from build123d import *

# Parameters (mm, degrees)
F0_R     = 10.9982
F1_DEPTH = 8.89


with BuildPart() as f1:
    # F0 (on Top) → F1 (new body)
    with BuildSketch(Plane.XY):
        with BuildLine():
            ThreePointArc((38.8529947684, 0), (28.4453239469, 28.4684513244), (0, 38.9391665957))
            ThreePointArc((0, 38.9391665957), (-27.8957339054, 28.0256688183), (-38.4710963646, 0))
            ThreePointArc((-38.4710963646, 0), (-27.9199689316, -27.9141662733), (0.0231951649, -38.3882556901))
            ThreePointArc((0.0231951649, -38.3882556901), (-9.5721699853, -15.3070070583), (13.5255, -24.8627755791))
            ThreePointArc((13.5255, -24.8627755791), (10.5110469105, -33.3749458719), (2.8113610633, -38.0928700316))
            ThreePointArc((2.8113610633, -38.0928700316), (29.4450372623, -27.1955065208), (38.8529947684, 0))
        make_face()
        with BuildLine():
            ThreePointArc((-11.4212829144, -0.1791534288), (-25.0363615935, -13.7043567881), (-38.4710963646, 0))
            ThreePointArc((-38.4710963646, 0), (-24.8572042354, 13.3460499305), (-11.4212829144, -0.1791534288))
        make_face(mode=Mode.SUBTRACT)
        Circle(F0_R, mode=Mode.SUBTRACT)
        with BuildLine():
            ThreePointArc((38.8531280306, 0.0600404714), (38.853094715, 0.0300201617), (38.8529947684, 0))
            ThreePointArc((38.8529947684, 0), (11.8021613462, 0.090060781), (38.8531280306, 0.0600404714))
        make_face(mode=Mode.SUBTRACT)
        with BuildLine():
            ThreePointArc((0, 38.9391665957), (9.8292581555, 34.8677545596), (13.9006701916, 25.0384964041))
            ThreePointArc((13.9006701916, 25.0384964041), (-9.8292581555, 15.2092382486), (0, 38.9391665957))
        make_face(mode=Mode.SUBTRACT)
        with BuildLine():
            ThreePointArc((0, 38.9391665957), (-9.8292581555, 15.2092382486), (13.9006701916, 25.0384964041))
            ThreePointArc((13.9006701916, 25.0384964041), (9.8292581555, 34.8677545596), (0, 38.9391665957))
        make_face()
        with Locations((0, 25.0384964041)):
            Circle(F0_R, mode=Mode.SUBTRACT)
        with BuildLine():
            ThreePointArc((-11.4212829144, -0.1791534288), (-24.8572042354, 13.3460499305), (-38.4710963646, 0))
            ThreePointArc((-38.4710963646, 0), (-25.0363615935, -13.7043567881), (-11.4212829144, -0.1791534288))
        make_face()
        with Locations((-24.9467829144, -0.1791534288)):
            Circle(F0_R, mode=Mode.SUBTRACT)
        with BuildLine():
            ThreePointArc((38.8531280306, 0.0600404714), (11.8021613462, 0.090060781), (38.8529947684, 0))
            ThreePointArc((38.8529947684, 0), (38.853094715, 0.0300201617), (38.8531280306, 0.0600404714))
        make_face()
        with Locations((25.3276280306, 0.0600404714)):
            Circle(F0_R, mode=Mode.SUBTRACT)
        with BuildLine():
            ThreePointArc((0.0231951649, -38.3882556901), (1.4201424448, -38.2675994791), (2.8113610633, -38.0928700316))
            ThreePointArc((2.8113610633, -38.0928700316), (10.5110469105, -33.3749458719), (13.5255, -24.8627755791))
            ThreePointArc((13.5255, -24.8627755791), (-9.5721699853, -15.3070070583), (0.0231951649, -38.3882556901))
        make_face()
        with Locations((0, -24.8627755791)):
            Circle(F0_R, mode=Mode.SUBTRACT)
        with BuildLine():
            ThreePointArc((0.0231951649, -38.3882556901), (1.4249527798, -38.3130045669), (2.8113610633, -38.0928700316))
            ThreePointArc((2.8113610633, -38.0928700316), (1.4201424448, -38.2675994791), (0.0231951649, -38.3882556901))
        make_face()
    extrude(amount=F1_DEPTH)


solid = f1.part
Can you work these out from the model? Positions are in its coordinate system, mm. Round coordinates to 2 decimals unless told otherwise and drop trailing zeros. Order: outer loops, then holes, each group sorted by start corner. A loop starts at its lowest first (then second) coordinate and runs counter-clockwise, first axis right, second up. Notation, with made-up numbers: M 36,17.5 L 93,17.5 A19 ccw 93,38.5 Z; hole C 29,63.5 d3. An arc over 180 degrees is marked long. Use a Markdown table: item, result.
1) If we mould it in two halves opening along X, with no side actions, what happens to faces 1 (the face through (5.075, -34.62, 4.383)), 2 (the face through (1.405, -38.315, 4.383)), 3 (the face through (8, -8, 0)), 4 (the face through (-14.787, -4.392, 4.383))? For each: +X half, -X half, draft (parallel to the pull), parting line (faces both ways), or undercut.
Geometry says:
| item | result |
|---|---|
| face 1 | undercut |
| face 2 | +X half |
| face 3 | draft |
| face 4 | undercut |
2) I'm going to push flat-ended pins straight in: P1, Ø1, axis at x = 25, z = 5.5, coming from the +Y side; P2, Ø1.5, axis at x = 26.5, z = 3.5, coming from the +Y side; P3, Ø5, axis at y = -24.5, z = 4, coming from the +X side. Where does each tip first touch, or does it pass through?
Geometry says:
| item | result |
|---|---|
| P1 | stops at y = 31.89 |
| P2 | stops at y = 30.91 |
| P3 | stops at x = 33.5 |
3) If I drill on line 1 along X through (y, z) = (-2, 5); line 2 along Y through (x, z) = (-5.5, 4); line 3 along X through (y, z) = (5, 0.5), over which ranges is the centre line in solid material (lowest first)?
Geometry says:
| item | result |
|---|---|
| line 1 | x = -38.54 to -35.79, -14.1 to -10.81, 10.81 to 14.52, 36.13 to 38.98 |
| line 2 | y = -38.33 to -34.39, -15.34 to -9.52, 9.52 to 15.51, 34.56 to 38.78 |
| line 3 | x = -38.42 to -34.65, -15.24 to -9.8, 9.8 to 15.5, 35.15 to 38.92 |
4) Imagine slicing it at A-A (x = 29). List the corners of the cut face in (y, z) for me.
Geometry says:
| item | result |
|---|---|
| outline | M -27.66,0 L -10.31,0 L -10.31,8.89 L -27.66,8.89 Z; M 10.43,0 L 27.9,0 L 27.9,8.89 L 10.43,8.89 Z |
5) Imagine slicing it at C-C (z = 3.25). List the corners of the cut face in (x, y) for me.
Geometry says:
| item | result |
|---|---|
| outline | M -38.47,0 A36.16 ccw 0.02,-38.39 A13.53 ccw 2.81,-38.09 A34.92 ccw 38.85,0 A36.06 ccw 0,38.94 A36.85 ccw Z; hole C -24.95,-0.18 d22; hole C 0,-24.86 d22; hole C 0,0 d22; hole C 0,25.04 d22; hole C 25.33,0.06 d22 |
6) Imagine slicing it at B-B (y = 2.5). List the corners of the cut face in (x, z) for me.
Geometry says:
| item | result |
|---|---|
| outline | M -38.53,0 L -35.61,0 L -35.61,8.89 L -38.53,8.89 Z; M -14.28,0 L -10.71,0 L -10.71,8.89 L -14.28,8.89 Z; M 10.71,0 L 14.6,0 L 14.6,8.89 L 10.71,8.89 Z; M 36.05,0 L 38.97,0 L 38.97,8.89 L 36.05,8.89 Z |
7) Imagine slicing it at D-D (x = 5.5). List the corners of the cut face in (y, z) for me, then the cut area to 3 significant figures.
Geometry says:
| item | result |
|---|---|
| outline | M -38.09,0 L -34.39,0 L -34.39,8.89 L -38.09,8.89 Z; M -15.34,0 L -9.52,0 L -9.52,8.89 L -15.34,8.89 Z; M 9.52,0 L 15.51,0 L 15.51,8.89 L 9.52,8.89 Z; M 34.56,0 L 38.97,0 L 38.97,8.89 L 34.56,8.89 Z |
| area | 177 mm² |
